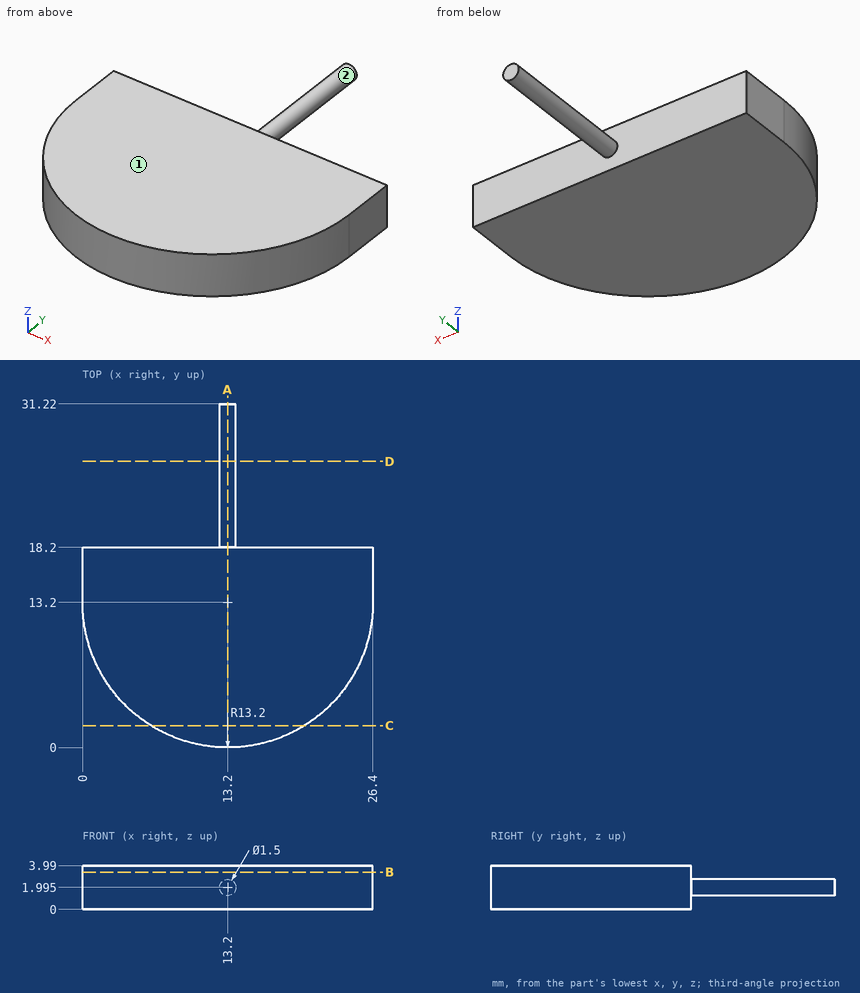
Input: dimensioned drawing with shaded views. Units: mm. Origin: part minimum x, y, z. A direction names the side the tool comes from. Give positions to 0.01 mm unless a question says otherwise; leave off trailing zeros. Write each loop counter-clockwise with the first axis right and the second up, starting at its lowest first coordinate (ties: lowest second). Pieces come first, ordered by that corner, then holes. Notation, with made-up numbers: (49.5, 87.25) -> (58.5, 87.25) arc R19 cw to (58.5, 124.25) -> close; hole circle Ø10 at (-35, 33.5). An arc over 180 degrees is marked (long way). Return JSON: item names as keys, results as strings. Group by question number.
1. Material intervals for line 1 (X direction, y = 21.5, z = 2); line 2 (X direction, y = 18.5, z = 1.5); line 3 (Y direction, x = 15.5, z = 1.45), sorted ascending. Write a range as from..to.
2. Section D-D, the plane y = 26. Output: boundary loops of the cut face in (x, z) (3 decimals), then the cut area to 3 significant figures.
3. Pin query (flat end, axial travel): pin 1 Ø1 at (x, z) = (4, 3) entering from -Y; pin 2 Ø2 at (x, z) = (9, 0.5) entering from -Y. Return the tip coordinate at first contact, or that it passes through.
4. Section B-B, the plane z = 3.4. Output: boundary loops of the cut face in (x, y).
5. Section C-C, the plane y = 2. Output: boundary loops of the cut face in (x, z), then the cut area to 3 significant figures.
6. Access query for the marked faces 1 and 2. Directions: +Z, -Z, +X, -X, +Y, -Y. A direction counts if a zero-diameter tool reaches every point of the face in a straight line with its end or side. Return the directions, or none.
7. Section A-A, the plane x = 13.2. Output: boundary loops of the cut face in (y, z) (3 decimals).
Determined:
{
 "1": {"line 1": "x = 12.45..13.95", "line 2": "x = 12.64..13.76", "line 3": "y = 0.2..18.2"},
 "2": {"outline": "circle Ø1.5 at (13.2, 1.995)", "area": "1.77 mm2"},
 "3": {"pin 1": "stops at y = 3.27", "pin 2": "stops at y = 0.39"},
 "4": {"outline": "(0, 13.2) arc R13.2 ccw to (26.4, 13.2) -> (26.4, 18.2) -> (0, 18.2) -> close"},
 "5": {"outline": "(6.21, 0) -> (20.19, 0) -> (20.19, 3.99) -> (6.21, 3.99) -> close", "area": "55.7 mm2"},
 "6": {"face 1": "+Z, +X, -X, +Y, -Y", "face 2": "+Y"},
 "7": {"outline": "(0, 0) -> (18.2, 0) -> (18.2, 1.245) -> (31.22, 1.245) -> (31.22, 2.745) -> (18.2, 2.745) -> (18.2, 3.99) -> (0, 3.99) -> close"}
}
